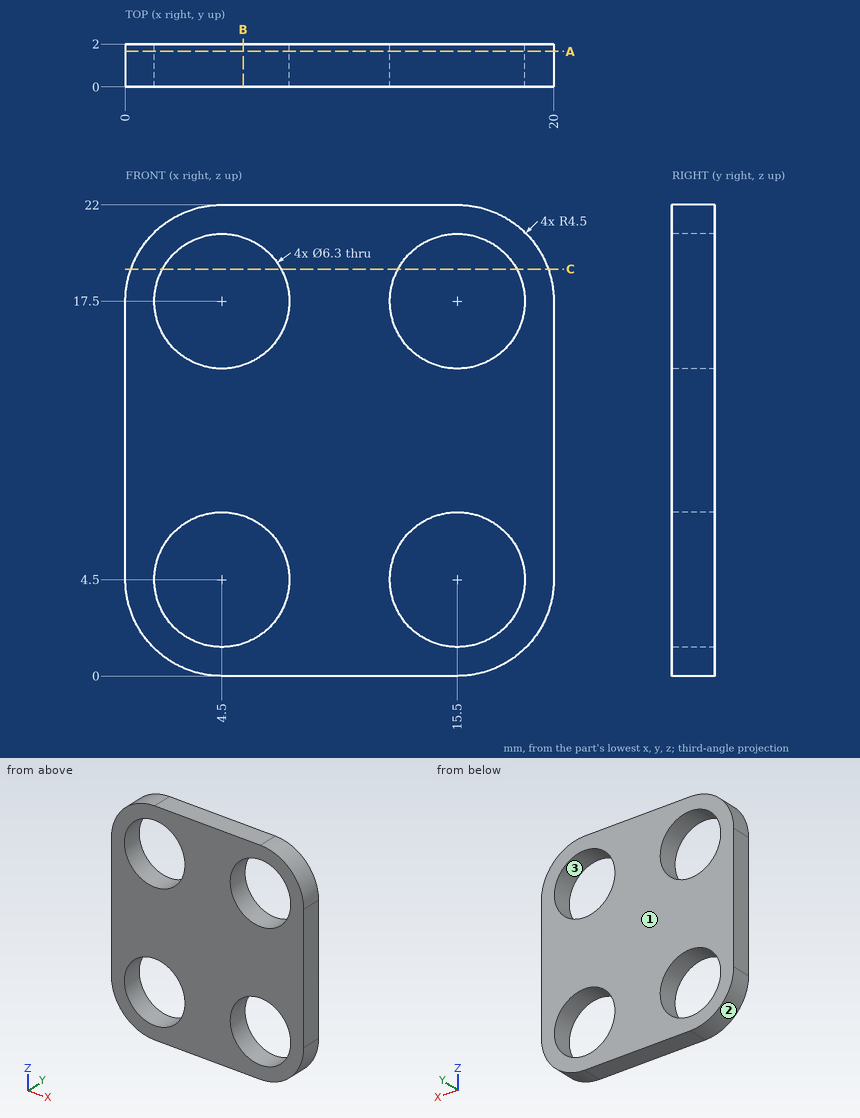
Input: dimensioned drawing with shaded views. Units: mm. Origin: part minimum x, y, z. Coordinates: 2 decimals unless noted, no trailing zeros. Order: outer loops, then holes, each group sorted by start corner. A loop starts at its lowest first (then second) coordinate and runs counter-clockwise, first axis right, second up. Notation, with made-up numbers: (34.5, 33.25) - (38.5, 33.25) arc R29 ccw to (38.5, 66.25) - close; hole circle Ø8 at (8.5, 52). An arc over 180 degrees is marked (long way). One line per item, written item: value.
1) Mould query, pull axis X, two halves, no side actions, for the marked faces 1, 2 and 3. Classes: released by +X, released by -X, zero draft, split by the parting line, or undercut.
Computed values:
face 1: zero draft
face 2: released by -X
face 3: undercut
2) Cut plane A-A on y = 1.65. Output: boundary loops of the cut face in (x, z), plus the area to 3 significant figures.
Computed values:
outline: (0, 4.5) arc R4.5 ccw to (4.5, 0) - (15.5, 0) arc R4.5 ccw to (20, 4.5) - (20, 17.5) arc R4.5 ccw to (15.5, 22) - (4.5, 22) arc R4.5 ccw to (0, 17.5) - close; hole circle Ø6.3 at (4.5, 4.5); hole circle Ø6.3 at (4.5, 17.5); hole circle Ø6.3 at (15.5, 4.5); hole circle Ø6.3 at (15.5, 17.5)
area: 298 mm^2
3) Contact query for flat-ended pins moving along their axis: pin 1 (7 mm diameter, centred on x = 4.5, z = 4.5, fed in from -Y); pin 2 (5 mm diameter, centred on x = 4.5, z = 17.5, fed in from +Y). Output: stop coordinate, or through.
Computed values:
pin 1: stops at y = 0
pin 2: passes through
4) Cut plane B-B on x = 5.5. Output: boundary loops of the cut face in (y, z).
Computed values:
outline: (0, 0) - (2, 0) - (2, 1.51) - (0, 1.51) - close; (0, 7.49) - (2, 7.49) - (2, 14.51) - (0, 14.51) - close; (0, 20.49) - (2, 20.49) - (2, 22) - (0, 22) - close
5) Ray query, line 1 (X direction, y = 1.1, z = 17.5); line 2 (Z direction, x = 15, y = 0.65); line 3 (Z direction, x = 13.25, y = 0.3). Return the intervals inside material, ascending. Write a range as [from, to].
Computed values:
line 1: x = [0, 1.35], [7.65, 12.35], [18.65, 20]
line 2: z = [0, 1.39], [7.61, 14.39], [20.61, 22]
line 3: z = [0, 2.3], [6.7, 15.3], [19.7, 22]
6) Cut plane C-C on z = 19. Output: boundary loops of the cut face in (x, y).
Computed values:
outline: (0.26, 0) - (1.73, 0) - (1.73, 2) - (0.26, 2) - close; (7.27, 0) - (12.73, 0) - (12.73, 2) - (7.27, 2) - close; (18.27, 0) - (19.74, 0) - (19.74, 2) - (18.27, 2) - close
